For this review, take the finished solid that the model builds, in its own axes (mm). Round coordinates to 2 decimals unless told otherwise and drop trailing zeros. Write each loop counter-clockwise with the first axis right and the second up, starting at its lowest first coordinate (ties: lowest second). Pieces come first, ordered by that corner, then holes. Notation, with made-up numbers: (17, 18) -> (67, 18) arc R26 ccw to (67, 49) -> close; hole circle Ø8 at (71.5, 67). An arc over 180 degrees is marked (long way). Answer in a Markdown table with one row per item.
from build123d import *

# Parameters (mm, degrees)
F0_R     = 2.38125
F1_DEPTH = 3.175
F2_R     = 6.35
F3_SIZE  = 1.27


with BuildPart() as f1:
    # F0 (on Top) → F1 (new body)
    with BuildSketch(Plane.XY):
        with BuildLine():
            Line((123.3248860695, 4.1671875), (3.6751139305, 4.1671875))
            ThreePointArc((3.6751139305, 4.1671875), (-5.55625, 0), (3.6751139305, -4.1671875))
            Line((3.6751139305, -4.1671875), (123.3248860695, -4.1671875))
            ThreePointArc((123.3248860695, -4.1671875), (127, -5.55625), (130.6751139305, -4.1671875))
            Line((130.6751139305, -4.1671875), (203.2, -4.1671875))
            Line((203.2, -4.1671875), (203.2, 4.1671875))
            Line((203.2, 4.1671875), (130.6751139305, 4.1671875))
            ThreePointArc((130.6751139305, 4.1671875), (127, 5.55625), (123.3248860695, 4.1671875))
        make_face()
        Circle(F0_R, mode=Mode.SUBTRACT)
        with Locations((127, 0)):
            Circle(F0_R, mode=Mode.SUBTRACT)
    extrude(amount=F1_DEPTH)

    # F2
    f2_edges = [f1.edges().sort_by_distance(p)[0] for p in [
        (3.675114, 4.167187, 1.5875),
        (3.675114, -4.167188, 1.5875),
        (123.324886, -4.167187, 1.5875),
        (130.675114, 4.167187, 1.5875),
        (123.324886, 4.167187, 1.5875),
        (130.675114, -4.167187, 1.5875),
    ]]
    fillet(f2_edges, radius=F2_R)

    # F3
    f3_edges = [f1.edges().sort_by_distance(p)[0] for p in [
        (63.5, 4.167187, 3.175),
        (63.5, 4.167187, 0),
        (127, 5.55625, 0),
        (127, 5.55625, 3.175),
        (131.047329, 4.355179, 0),
        (122.952671, 4.355179, 0),
        (167.8905, 4.167187, 0),
        (4.047329, 4.355179, 0),
        (167.8905, -4.167187, 0),
        (-5.55625, 0, 0),
        (131.047329, -4.355179, 0),
        (4.047329, -4.355179, 0),
        (127, -5.55625, 0),
        (63.5, -4.167187, 0),
        (122.952671, -4.355179, 0),
        (131.047329, 4.355179, 3.175),
        (122.952671, 4.355179, 3.175),
        (167.8905, 4.167187, 3.175),
        (4.047329, 4.355179, 3.175),
        (167.8905, -4.167187, 3.175),
        (-5.55625, 0, 3.175),
        (131.047329, -4.355179, 3.175),
        (4.047329, -4.355179, 3.175),
        (127, -5.55625, 3.175),
        (63.5, -4.167187, 3.175),
        (122.952671, -4.355179, 3.175),
    ]]
    chamfer(f3_edges, length=F3_SIZE)


solid = f1.part
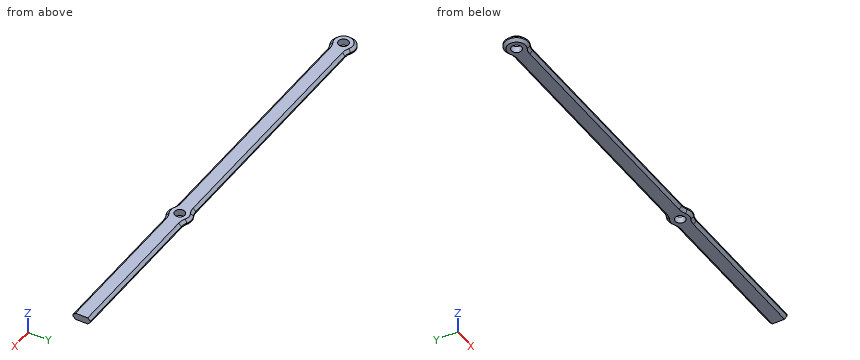
1) Consider section B-B on x = 0. State the section outline as (y, z) points (3 decimals), then the cut area to 3 significant figures.
Solved:
| item | result |
|---|---|
| outline | (-5.556, 1.27) -> (-4.286, 0) -> (-2.381, 0) -> (-2.381, 3.175) -> (-4.286, 3.175) -> (-5.556, 1.905) -> close; (2.381, 0) -> (4.286, 0) -> (5.556, 1.27) -> (5.556, 1.905) -> (4.286, 3.175) -> (2.381, 3.175) -> close |
| area | 16.9 mm² |
2) For line 1 (Y direction, x = 0, z = 1.45); line 2 (X direction, y = -5, z = 1.4); line 3 (X direction, y = -1.25, z = 2.65), list the stretches that pass through material, from the lowest coordinate up. Write a range as [from, to].
Solved:
| item | result |
|---|---|
| line 1 | [-5.56, -2.38], [2.38, 5.56] |
| line 2 | [-2.42, 2.42], [124.58, 129.42] |
| line 3 | [-4.65, -2.03], [2.03, 124.97], [129.03, 203.2] |
3) Clearance check with flat-ended pins moving along their axes: pin 1 Ø1.5 at (x, z) = (50, 2) entering from +Y; pin 2 Ø0.7 at (x, z) = (71.5, 1.5) entering from -Y; pin 3 Ø4.5 at (x, y) = (0, 0) entering from +Z. State where each tip first meets the part, or that it passes through.
Solved:
| item | result |
|---|---|
| pin 1 | y = 4.17 |
| pin 2 | y = -4.17 |
| pin 3 | through |
4) Consider section A-A on y = 0. State the section outline as (x, z) points (3 decimals).
Solved:
| item | result |
|---|---|
| outline | (-5.556, 1.27) -> (-4.286, 0) -> (-2.381, 0) -> (-2.381, 3.175) -> (-4.286, 3.175) -> (-5.556, 1.905) -> close; (2.381, 0) -> (124.619, 0) -> (124.619, 3.175) -> (2.381, 3.175) -> close; (129.381, 0) -> (203.2, 0) -> (203.2, 3.175) -> (129.381, 3.175) -> close |
5) Consider section C-C on x = 54.5. State the section outline as (y, z) points (3 decimals), then the cut area to 3 significant figures.
Solved:
| item | result |
|---|---|
| outline | (-4.167, 1.27) -> (-2.897, 0) -> (2.897, 0) -> (4.167, 1.27) -> (4.167, 1.905) -> (2.897, 3.175) -> (-2.897, 3.175) -> (-4.167, 1.905) -> close |
| area | 23.2 mm² |
6) Consider section D-D on z = 0.55. State the section outline as (x, y) points, then the cut area to 3 significant figures.
Solved:
| item | result |
|---|---|
| outline | (2.27, -4.27) arc R7.07 cw to (5.58, -3.45) -> (121.42, -3.45) arc R7.07 cw to (124.73, -4.27) arc R4.84 ccw to (129.27, -4.27) arc R7.07 cw to (132.58, -3.45) -> (203.2, -3.45) -> (203.2, 3.45) -> (132.58, 3.45) arc R7.07 cw to (129.27, 4.27) arc R4.84 ccw to (124.73, 4.27) arc R7.07 cw to (121.42, 3.45) -> (5.58, 3.45) arc R7.07 cw to (2.27, 4.27) arc R4.84 ccw (long way) to start; hole circle Ø4.76 at (0, 0); hole circle Ø4.76 at (127, 0) |
| area | 1,420 mm² |
